Here's how the part is built. I have some questions about the finished solid (model axes, mm). Face numbers are marked on the shaded views. A direction names the side the tool comes from. Coordinates: 2 decimals unless noted, no trailing zeros. Write each loop counter-clockwise with the first axis right and the second up, starting at its lowest first coordinate (ties: lowest second). Pieces come first, ordered by that corner, then holes.
(1) Thinking about a two-plate mould opening in Y: for the marked faces 5 and 6, which applies, released by +Y, released by -Y, zero draft, split by the parting line, or undercut?
(2) For pin 1 Ø2 at (x, z) = (9, -3) entering from +Y; pin 2 Ø4.5 at (y, z) = (3, -0.5) entering from -X; pin 3 Ø8 at (x, y) = (2, -2.5) entering from +Z, each with a flat end and sliding along its axis, tell me the tip position at first contact or that it passes through.
(3) Imagine slicing it at C-C, the plane x = 10.75. List the corners of the cut face in (y, z) for me, plus the area to 3 significant figures.
(4) Please list where these lines run through material, in increasing order: probe 1 along X at (y, z) = (-5.75, 4); probe 2 along X at (y, z) = (5.25, 14); probe 3 along Z at (x, y) = (-11.25, -6.5).
(5) Imagine slicing it at A-A, the plane y = 0. List the corners of the cut face in (x, z) for me.
(6) Imagine slicing it at D-D, the plane z = 8.25. List the corners of the cut face in (x, y) for me.
(7) Imagine slicing it at B-B, the plane x = 0. List the corners of the cut face in (y, z) for me, plus the area to 3 significant figures.
(8) Which directions (+Z, -Z, +X, -X, +Y, -Y) give clear straight access to the entire face, cutting with the end or side of a thin tool? Please do the marked faces 1, 2, 3 and 4.
```python
from build123d import *

# Parameters (mm, degrees)
F4_R     = 7.75
F5_DEPTH = 6
F6_R     = 7.75
F7_DEPTH = 6


# Not quite as in the source:
# - a pattern or mirror of a feature is missing from the dataset's text; its kind, count and spacing are read off the source's solid


with BuildPart() as f1:
    # F0 (on Front) → F1 (revolve)
    with BuildSketch(Plane.XZ):
        Polygon((13.5, 9.25), (0, 9.25), (-13.5, 9.25), (-13.5, 0), (0, 0), (13.5, 0), align=None)
    revolve(axis=Axis((6.75, 0, 0), (-1, 0, 0)))

    # F2 (on Front) → F3 (revolve)
    with BuildSketch(Plane.XZ):
        Polygon((9.25, 19.0967741935), (0, 19.0967741935), (0, 8.3548387097), (0, 0), (9.25, 0), (9.25, 8.3548387097), align=None)
    revolve(axis=Axis((0, 0, 13.7258064516), (0, 0, 1)))

    # F4 (on face) → F5 (cut)
    with BuildSketch(Plane.YZ.offset(13.5)):
        Circle(F4_R)
    f5 = extrude(amount=-F5_DEPTH, mode=Mode.SUBTRACT)

    # F5_copies: F5 across plane
    add(f5.mirror(Plane(origin=(0, 0, 0), x_dir=(0, 0, -1), z_dir=(-1, 0, 0))), mode=Mode.SUBTRACT)

    # F6 (on face) → F7 (cut)
    with BuildSketch(Plane.XY.offset(19.0967741935)):
        Circle(F6_R)
    extrude(amount=-F7_DEPTH, mode=Mode.SUBTRACT)


solid = f1.part
```
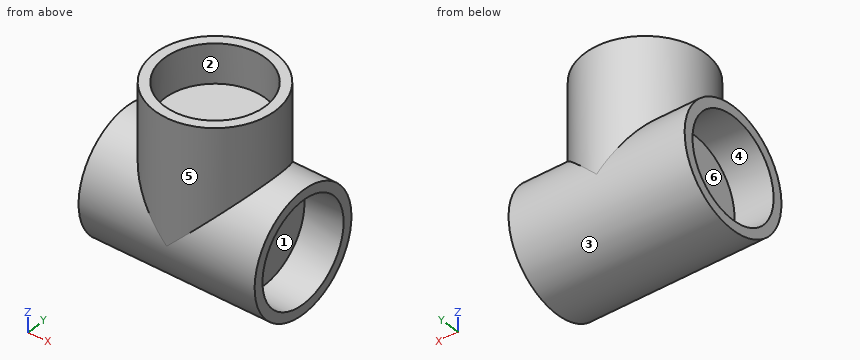
Recorded:
1. face 5: split by the parting line
1. face 6: undercut
2. pin 1: stops at y = 9.03
2. pin 2: stops at x = -7.5
2. pin 3: stops at z = 13.1
3. outline: circle Ø18.5 at (0, 0); hole circle Ø15.5 at (0, 0)
3. area: 80.1 mm2
4. probe 1: x = -7.5 to 7.5
4. probe 2: x = -7.62 to -5.7, 5.7 to 7.62
4. probe 3: z = -6.58 to -4.22, 4.22 to 6.58
5. outline: (-13.5, -9.25) - (13.5, -9.25) - (13.5, -7.75) - (7.5, -7.75) - (7.5, 7.75) - (13.5, 7.75) - (13.5, 9.25) - (9.25, 9.25) - (9.25, 19.1) - (7.75, 19.1) - (7.75, 13.1) - (-7.75, 13.1) - (-7.75, 19.1) - (-9.25, 19.1) - (-9.25, 9.25) - (-13.5, 9.25) - (-13.5, 7.75) - (-7.5, 7.75) - (-7.5, -7.75) - (-13.5, -7.75) - close
6. outline: (-13.5, -4.18) - (-8.25, -4.18) arc R9.25 ccw to (8.25, -4.18) - (13.5, -4.18) - (13.5, 4.18) - (8.25, 4.18) arc R9.25 ccw to (-8.25, 4.18) - (-13.5, 4.18) - close
7. outline: (-9.25, 0) arc R9.25 ccw to (9.25, 0) - (9.25, 19.1) - (7.75, 19.1) - (7.75, 13.1) - (-7.75, 13.1) - (-7.75, 19.1) - (-9.25, 19.1) - close
7. area: 395 mm2
8. face 1: +X
8. face 2: +Z
8. face 3: none
8. face 4: -X
